Geometry: see drawing. Coordinates: mm, zero at the bounding-box minimum. Give positions to 0.01 mm unless a question says otherwise; leave off trailing zeros. Write each loop counter-clockwise with the first axis right and the second up, starting at its lowest first coordinate (ties: lowest second). Pieces come first, ordered by that corner, then holes. Notation, with made-up numbers: (-2.75, 66.25) -> (37.25, 66.25) arc R5 cw to (37.25, 71.25) -> close; hole circle Ø3 at (26, 13). An arc over 180 degrees is marked (long way). Use one line per item in the form item = value. Start each with the question number.
(1) Cut plane B-B, the plane z = 2.75. Output: boundary loops of the cut face in (x, y).
(2) Material intervals for line 1 along Y through (x, z) = (38.1, 7); line 2 along Z through (x, y) = (19.05, 9.75); line 3 along X through (y, z) = (64, 9) (1 decimal), sorted ascending. Write a range as from..to.
(3) First-contact query: P1, Ø1.5, axis at x = 61.5, z = 10, coming from the +Y side; P2, Ø1.5, axis at x = 9.5, z = 8, coming from the +Y side; P3, Ø2, axis at x = 67, z = 5.5, coming from the +Y side. Flat tips, straight axial feed; report the tip coordinate or a pass-through.
(4) Draft query along Y for the marked faces 1, 2 and 3. Return one class per face: pulls with the +Y half, pulls with the -Y half, needs draft (parallel to the pull), parting line crosses it, or undercut.
(5) Cut plane A-A, the plane x = 38.1. Output: boundary loops of the cut face in (y, z).
(6) Cut plane C-C, the plane y = 44.45. Output: boundary loops of the cut face in (x, z).
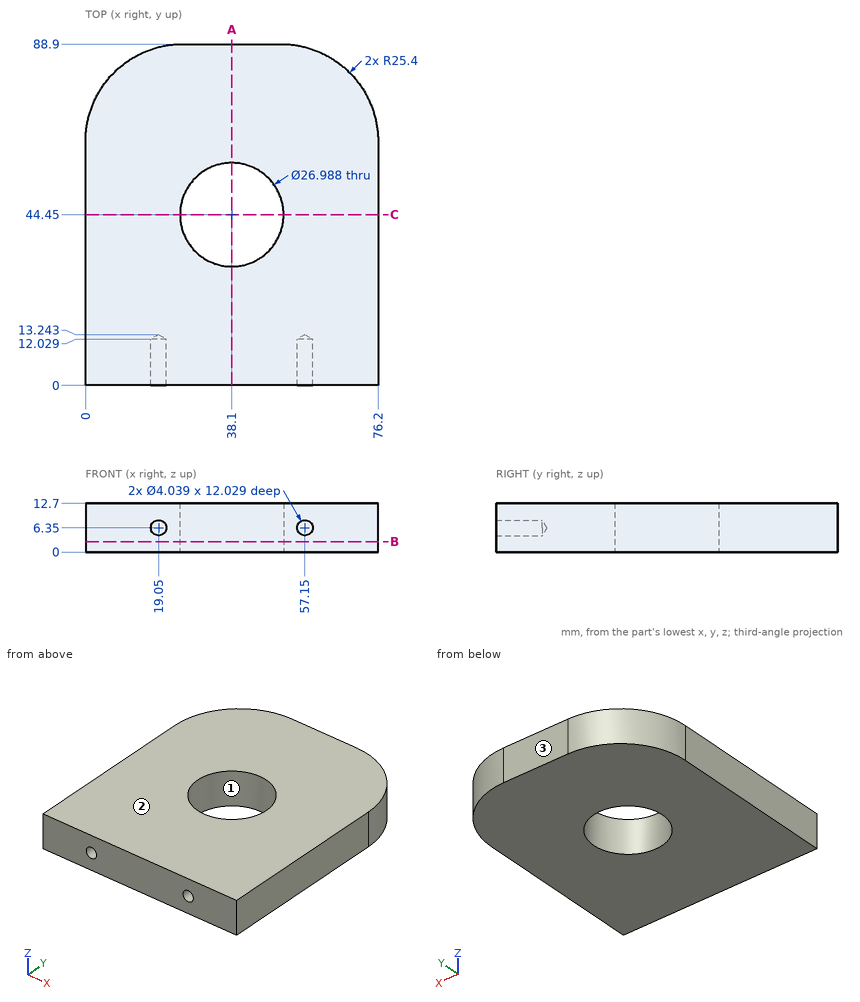
Geometry says:
q1.outline = (0, 0) -> (76.2, 0) -> (76.2, 63.5) arc R25.4 ccw to (50.8, 88.9) -> (25.4, 88.9) arc R25.4 ccw to (0, 63.5) -> close; hole circle Ø26.99 at (38.1, 44.45)
q2.line_1 = 0..30.96, 57.94..88.9
q2.line_2 = 0..4.33, 8.37..12.7
q2.line_3 = 0..76.2
q3.P1 = 86.87
q3.P2 = 83.89
q3.P3 = 83.85
q4.face_1 = undercut
q4.face_2 = needs draft
q4.face_3 = pulls with the +Y half
q5.outline = (0, 0) -> (30.96, 0) -> (30.96, 12.7) -> (0, 12.7) -> close; (57.94, 0) -> (88.9, 0) -> (88.9, 12.7) -> (57.94, 12.7) -> close
q6.outline = (0, 0) -> (24.61, 0) -> (24.61, 12.7) -> (0, 12.7) -> close; (51.59, 0) -> (76.2, 0) -> (76.2, 12.7) -> (51.59, 12.7) -> close
